The listing builds one solid part. Answer for the finished solid, in the listing's coordinates (mm). Face numbers are marked on the shaded views. A direction names the side the tool comes from. Give positions to 0.01 mm unless a question says otherwise; leave off trailing zeros. Loops run counter-clockwise (first coordinate to the right, second up) from the corner with the lowest first, then second, coordinate; pieces in that order, holes last.
Item 1: Section A-A, the plane y = 10.45 is taken. Give the vertices of the cut face in (x, z).
Item 2: The mould has two halves that part along X. Classify the marked faces 1, 2 and 3: pulls with the +X half, pulls with the -X half, needs draft (parallel to the pull), parting line crosses it, or undercut.
Item 3: Each of these flat-tipped pins is pushed along its axis until it touches: pin 1 Ø2.5 at (x, z) = (45, 10) entering from +Y; pin 2 Ø5 at (x, z) = (-24, 12) entering from -Y; pin 3 Ø2 at (y, z) = (42, 13) entering from -X. Where does it stop, or does it pass through?
Item 4: Section C-C, the plane x = 44.1 is taken. Give the vertices of the cut face in (y, z) (3 decimals).
Item 5: Section B-B, the plane y = -2.5 is taken. Give the vertices of the cut face in (x, z), and give its area (3 significant figures).
Item 6: Section D-D, the plane z = 16.5 is taken. Give the vertices of the cut face in (x, y).
Item 7: Consider line 1 along X through (y, z) = (17, 16.25); line 2 along Y through (x, z) = (67.25, 10); line 3 along Z through (x, y) = (-44.1, 43.75) (3 decimals). Determine where each line is inside the solid, lowest interval first.
Item 8: A tool of negligible diameter and unlimited length cuts with its end or side. For the marked faces 4, 5 and 6, from which of +Z, -Z, +X, -X, +Y, -Y can it reach the whole face along a straight path? Write none if from no direction.
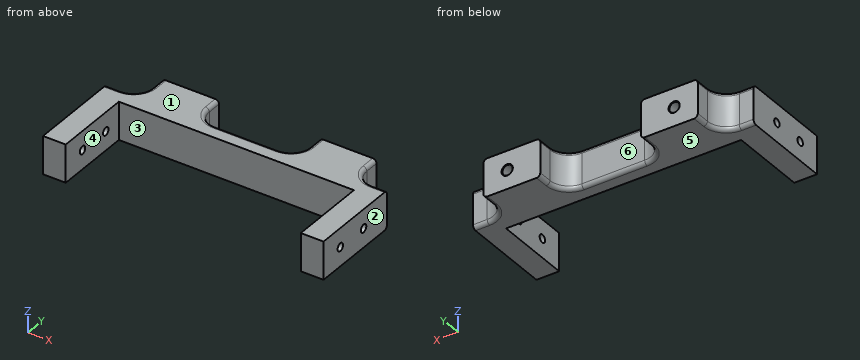
from build123d import *

# Parameters (mm, degrees)
BOSS_EXTRUDE1_DEPTH  = 20
SKETCH2_R            = 2.1
CUT_EXTRUDE1_DEPTH   = 149
SKETCH3_W            = 30
SKETCH3_H            = 17.5
BOSS_EXTRUDE2_DEPTH  = 20
FILLET1_R            = 10
FILLET1_OF_MIRROR1_R = 10
FILLET2_R            = 2
SKETCH4_R            = 2.675
CUT_EXTRUDE2_DEPTH   = 7
CHAMFER1_SIZE        = 0.3


with BuildPart() as part:
    # Sketch1 → Boss-Extrude1 (new body)
    with BuildSketch(Plane.XY):
        Polygon((-74.1, 28.55), (-74.1, -20.55), (-62.1, -20.55), (-62.1, 20.55), (62.1, 20.55), (62.1, -20.55), (74.1, -20.55), (74.1, 28.55), align=None)
    extrude(amount=BOSS_EXTRUDE1_DEPTH)

    # Sketch2 → Cut-Extrude1 (cut)
    with BuildSketch(Plane.ZY.offset(74.1)):
        with Locations((10, 10.45)):
            Circle(SKETCH2_R)
        with Locations((10, -7.55)):
            Circle(SKETCH2_R)
    extrude(amount=-CUT_EXTRUDE1_DEPTH, mode=Mode.SUBTRACT)

    # Sketch3 → Boss-Extrude2 (add)
    with BuildSketch(Plane.XY.offset(20)):
        with Locations((-41.6, 37.3)):
            Rectangle(SKETCH3_W, SKETCH3_H)
    boss_extrude2 = extrude(amount=-BOSS_EXTRUDE2_DEPTH)

    # Fillet1
    fillet1_edges = [part.edges().sort_by_distance(p)[0] for p in [
        (-26.6, 28.55, 10),
        (-56.6, 28.55, 10),
    ]]
    fillet(fillet1_edges, radius=FILLET1_R)

    # Mirror1: Boss-Extrude2 across plane
    add(boss_extrude2.mirror(Plane(origin=(0, 0, 0), x_dir=(0, 0, 1), z_dir=(1, 0, 0))))

    # Fillet1 of Mirror1
    fillet1_of_mirror1_edges = [part.edges().sort_by_distance(p)[0] for p in [
        (26.6, 28.55, 10),
        (56.6, 28.55, 10),
    ]]
    fillet(fillet1_of_mirror1_edges, radius=FILLET1_OF_MIRROR1_R)

    # Fillet2
    fillet2_edges = [part.edges().sort_by_distance(p)[0] for p in [
        (70.35, 28.55, 20),
        (-56.6, 42.3, 0),
        (-56.6, 42.3, 20),
        (-26.6, 42.3, 20),
        (-26.6, 42.3, 0),
        (-70.35, 28.55, 0),
        (-70.35, 28.55, 20),
        (-23.671067812, 31.478932188, 20),
        (-23.671067812, 31.478932188, 0),
        (-59.528932188, 31.478932188, 20),
        (-59.528932188, 31.478932188, 0),
        (56.6, 42.3, 20),
        (56.6, 42.3, 0),
        (26.6, 42.3, 20),
        (26.6, 42.3, 0),
        (0, 28.55, 0),
        (0, 28.55, 20),
        (23.671067812, 31.478932188, 20),
        (23.671067812, 31.478932188, 0),
        (59.528932188, 31.478932188, 20),
        (59.528932188, 31.478932188, 0),
        (70.35, 28.55, 0),
    ]]
    fillet(fillet2_edges, radius=FILLET2_R)

    # Sketch4 → Cut-Extrude2 (cut)
    with BuildSketch(Plane(origin=(0, 46.05, 0), x_dir=(1, 0, 0), z_dir=(0, 1, 0))):
        with Locations(Location((44.1, -10, 0), (0, 0, 180))):
            Circle(SKETCH4_R)
        with Locations(Location((-44.1, -10, 0), (0, 0, 180))):
            Circle(SKETCH4_R)
    extrude(amount=-CUT_EXTRUDE2_DEPTH, mode=Mode.SUBTRACT)

    # Chamfer1
    chamfer1_edges = [part.edges().sort_by_distance(p)[0] for p in [
        (46.775, 46.05, 10),
        (-41.425, 46.05, 10),
    ]]
    chamfer(chamfer1_edges, length=CHAMFER1_SIZE)


solid = part.part
Worked answers:
1. outline: (-74.1, 0) - (-62.1, 0) - (-62.1, 7.9) - (-74.1, 7.9) - close; (-74.1, 12.1) - (-62.1, 12.1) - (-62.1, 20) - (-74.1, 20) - close; (62.1, 0) - (74.1, 0) - (74.1, 7.9) - (62.1, 7.9) - close; (62.1, 12.1) - (74.1, 12.1) - (74.1, 20) - (62.1, 20) - close
2. face 1: needs draft
2. face 2: pulls with the +X half
2. face 3: undercut
3. pin 1: stops at y = 39.05
3. pin 2: stops at y = 20.55
3. pin 3: stops at x = -56.6
4. outline: (20.55, 0) - (46.05, 0) - (46.05, 7.025) - (45.75, 7.325) - (39.05, 7.325) - (39.05, 12.675) - (45.75, 12.675) - (46.05, 12.975) - (46.05, 20) - (20.55, 20) - close
5. outline: (-74.1, 0) - (-62.1, 0) - (-62.1, 20) - (-74.1, 20) - close; (62.1, 0) - (74.1, 0) - (74.1, 20) - (62.1, 20) - close
5. area: 480 mm2
6. outline: (-74.1, -20.55) - (-62.1, -20.55) - (-62.1, 20.55) - (62.1, 20.55) - (62.1, -20.55) - (74.1, -20.55) - (74.1, 28.55) - (66.6, 28.55) arc R10 cw to (56.6, 38.55) - (56.6, 46.05) - (26.6, 46.05) - (26.6, 38.55) arc R10 cw to (16.6, 28.55) - (-16.6, 28.55) arc R10 cw to (-26.6, 38.55) - (-26.6, 46.05) - (-56.6, 46.05) - (-56.6, 38.55) arc R10 cw to (-66.6, 28.55) - (-74.1, 28.55) - close
7. line 1: x = -74.1 to -62.1, 62.1 to 74.1
7. line 2: y = -20.55 to -9.65, -5.45 to 8.35, 12.55 to 28.55
7. line 3: z = 0 to 7.325, 12.675 to 20
8. face 4: +Z, -Z, -Y
8. face 5: -Z, +X, -X, +Y, -Y
8. face 6: +Z, -Z, +Y
